Model file for the job. Use its own axes, mm. Face numbers are marked on the shaded views. A direction names the side the tool comes from. Coordinates: 2 decimals unless noted, no trailing zeros. Write each loop counter-clockwise with the first axis right and the second up, starting at its lowest first coordinate (ties: lowest second). Pieces come first, ordered by that corner, then holes. Notation, with made-up numbers: M -4.75,14 L 45.25,14 A11 ccw 45.25,31 Z; hole C 82.5,54 d8. An arc over 180 degrees is marked long. One line per question, with ' | ' between items. Start each with the question number.
(1) Wall check: probe 1 along X at (y, z) = (6, 15); probe 2 along Z at (x, y) = (-30.5, 28.5); probe 3 along X at (y, z) = (1.5, 34). Give the ranges that are in metal, low to high.
(2) Two-plate mould, pull along X, no slides. Class the marked faces 1, 2, 3 and 4: +X half, -X half, draft (parallel to the pull), parting line (faces both ways), or undercut.
(3) Cut at B-B (y = 22). Write the cut outline in (x, z).
(4) Tool access for the marked faces 5, 6 and 7: list every direction of +Z, -Z, +X, -X, +Y, -Y with a clear straight run to the whole face (end or side of a thin tool).
(5) Cut at A-A (z = 18.5). Write the cut outline in (x, y), plus the area to 3 significant figures.
(6) Flat gauge pins, fed straight in: pin 1 Ø12 at (x, y) = (-75.5, 17.5) entering from +Z; pin 2 Ø14 at (y, z) = (15, 26.5) entering from +X; pin 3 Ø12 at (x, z) = (-77.5, 8.5) entering from -Y; pin 4 Ø4 at (x, y) = (-39.34, 12.21) entering from +Z. Where does each tip first touch, or does it go through?
from build123d import *

# Parameters (mm, degrees)
F1_DEPTH = 35
F0_W     = 3
F0_H     = 37
F0_R     = 2.5
F0_W_2   = 37
F2_DEPTH = 5
F3_R     = 2
F4_SIZE  = 3
F5_R     = 1
F6_SIZE  = 2
F7_R     = 2
F9_DEPTH = 12.5


# Not quite as in the source:
# - a fillet or chamfer that OpenCascade refuses, or shapes differently, is made with other operations: its cross-section is extruded or revolved along the edge and cut away or added
# - a feature names something its author has since deleted; it is built from what else it names


with BuildPart() as f1:
    # F0 (on Top) → F1 (new body)
    with BuildSketch(Plane.XY):
        Polygon((-89.3438757165, 12.2090974661), (-89.3438757165, 30.7090974661), (-95.3438757165, 30.7090974661), (-95.3438757165, -6.2909025339), (-89.3438757165, -6.2909025339), align=None)
    extrude(amount=F1_DEPTH)



with BuildPart() as f1b:
    # F0 (on Top) → F1, piece 2 (new body)
    with BuildSketch(Plane.XY):
        with Locations((-49.8438757165, 12.2090974661)):
            Rectangle(F0_W, F0_H)
    extrude(amount=F1_DEPTH)


with BuildPart() as f1_1:
    add(f1.part)

    add(f1b.part)  # F2 merges F1b
    # F0 (on Top) → F2 (join)
    with BuildSketch(Plane.XY):
        Polygon((-51.3438757165, 30.7090974661), (-89.3438757165, 30.7090974661), (-89.3438757165, 12.2090974661), (-89.3438757165, -6.2909025339), (-51.3438757165, -6.2909025339), align=None)
        with Locations((-77.8438757165, 12.2090974661)):
            Circle(F0_R, mode=Mode.SUBTRACT)
        with BuildLine():
            ThreePointArc((-65.3438757165, 12.2090974661), (-62.8438757165, 14.7090974661), (-60.3438757165, 12.2090974661))
            ThreePointArc((-60.3438757165, 12.2090974661), (-62.8438757165, 9.7090974661), (-65.3438757165, 12.2090974661))
        make_face(mode=Mode.SUBTRACT)
        with Locations((-29.8438757165, 12.2090974661)):
            Rectangle(F0_W_2, F0_H)
        with Locations((-39.3354164958, 12.2090974661)):
            Circle(F0_R, mode=Mode.SUBTRACT)
        with Locations((-20.3354164958, 12.2090974661)):
            Circle(F0_R, mode=Mode.SUBTRACT)
    extrude(amount=F2_DEPTH)

    # F3
    f3_edges = [f1_1.edges().sort_by_distance(p)[0] for p in [
        (-89.343876, 12.209097, 5),
        (-51.343876, 12.209097, 5),
        (-48.343876, 12.209097, 35),
    ]]
    fillet(f3_edges, radius=F3_R)

    # F4
    f4_edges = [f1_1.edges().sort_by_distance(p)[0] for p in [
        (-11.343876, 12.209097, 0),
    ]]
    chamfer(f4_edges, length=F4_SIZE)

    # F5
    f5_edges = [f1_1.edges().sort_by_distance(p)[0] for p in [
        (-11.343876, 12.209097, 3),
    ]]
    fillet(f5_edges, radius=F5_R)

    # F6
    f6_edges = [f1_1.edges().sort_by_distance(p)[0] for p in [
        (-65.343876, 12.209097, 0),
        (-41.835416, 12.209097, 0),
        (-22.835416, 12.209097, 0),
        (-80.343876, 12.209097, 0),
    ]]
    chamfer(f6_edges, length=F6_SIZE)

    # F7
    f7_edges = [f1_1.edges().sort_by_distance(p)[0] for p in [
        (-95.343876, 12.209097, 35),
        (-95.343876, 12.209097, 0),
    ]]
    fillet(f7_edges, radius=F7_R)

    # F8 (on face) → F9 (cut, symmetric)
    with BuildSketch(Plane(origin=(-95.3438757165, 0, 0), x_dir=(0, -1, 0), z_dir=(-1, 0, 0))):
        with BuildLine():
            ThreePointArc((-9.7090974661, 28.8686309451), (-10.4413305132, 30.636397898), (-12.2090974661, 31.3686309451))
            Line((-12.2090974661, 31.3686309451), (-12.2090974661, 26.3686309451))
            ThreePointArc((-12.2090974661, 26.3686309451), (-10.4413305132, 27.1008639921), (-9.7090974661, 28.8686309451))
        make_face()
        with BuildLine():
            Line((-12.2090974661, 26.3686309451), (-12.2090974661, 31.3686309451))
            ThreePointArc((-12.2090974661, 31.3686309451), (-14.7090974661, 28.8686309451), (-12.2090974661, 26.3686309451))
        make_face()
    extrude(amount=F9_DEPTH, both=True, mode=Mode.SUBTRACT)

    # F10: chamfer of 2 on 1 edges, made by hand

    # F10_s1 → F10_t2 (revolve, cut)
    with BuildSketch(Plane.XY.offset(28.8686309451)):
        Polygon((-95.3438757165, 7.7090974661), (-93.3438757165, 9.7090974661), (-95.3438757165, 9.7090974661), align=None)
    revolve(axis=Axis((-95.3438757165, 12.2090974661, 28.8686309451), (-1, 0, 0)), mode=Mode.SUBTRACT)


solid = f1_1.part
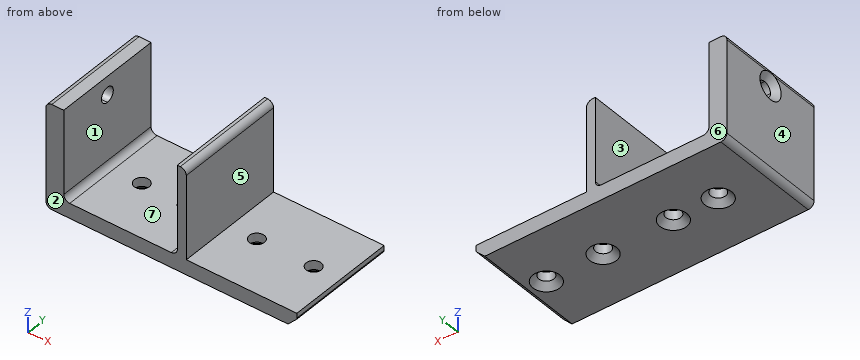
Filled in:
1) probe 1: -95.34 to -89.34, -51.34 to -48.34 | probe 2: 0 to 5 | probe 3: -95.08 to -89.34, -51.34 to -48.61
2) face 1: undercut | face 2: draft | face 3: undercut | face 4: -X half
3) outline: M -95.34,2 A2 ccw -93.34,0 L -14.34,0 L -11.64,2.71 A1 ccw -11.34,3.41 L -11.34,5 L -48.34,5 L -48.34,33 A2 ccw -50.34,35 L -51.34,35 L -51.34,7 A2 cw -53.34,5 L -87.34,5 A2 cw -89.34,7 L -89.34,35 L -93.34,35 A2 ccw -95.34,33 Z
4) face 5: +Z, +X, +Y, -Y | face 6: +Z, -Z, +X, -X, +Y | face 7: +Z, +Y, -Y
5) outline: M -95.34,-6.29 L -89.34,-6.29 L -89.34,30.71 L -95.34,30.71 Z; M -51.34,-6.29 L -48.34,-6.29 L -48.34,30.71 L -51.34,30.71 Z | area: 333 mm²
6) pin 1: z = 5 | pin 2: x = -48.34 | pin 3: y = -6.29 | pin 4: through
